The figure shows three views and two pictorial views of one solid part (mm, origin at its lowest corner). Answer the questions. A direction names the side the tool comes from. Round coordinates to 2 decimals unless told otherwise and drop trailing zeros. Write each loop counter-clockwise with the first axis right and the second up, starting at its lowest first coordinate (ties: lowest second). Pieces come first, ordered by that corner, then holes. Notation, with made-up numbers: (44.25, 57.25) - (60.25, 57.25) arc R23 cw to (60.25, 91.25) - close; hole circle Ø3 at (21, 4.5). An arc over 180 degrees is marked (long way). Answer as CSV lines item,"result". Start each with the question number.
Item 1: Which of the six approach directions +Z, -Z, +X, -X, +Y, -Y give full straight-line access (tool end or side, diameter ignored) to the marked faces 1, 2 and 3?
Item 2: For a pull along X with two mould halves and no side action, classify the marked faces 4, 5 and 6 as pulls with the +X half, pulls with the -X half, needs draft (parallel to the pull), parting line crosses it, or undercut.
Item 3: A cutting plane is placed at A-A on z = 3. Determine the outline of the cut face in (x, y).
Item 4: A cutting plane is placed at D-D on z = 0.95. Determine the outline of the cut face in (x, y), and give its area (3 significant figures).
Item 5: Straight lines are drawn through the part: line 1 along X through (y, z) = (15, 1.4); line 2 along X through (y, z) = (15, 2.95); line 3 along Y through (x, z) = (19, 3.2). For each, find the intervals that lie inside material, in ascending order. Write a range as [from, to].
Item 6: A cutting plane is placed at C-C on y = 15. Determine the outline of the cut face in (x, z).
Item 7: Flat-ended cylindrical pins translate along their axes: pin 1 (1 mm diameter, centred on y = 3.5, z = 3.5, fed in from +X); pin 2 (1.7 mm diameter, centred on x = 18, y = 15.5, fed in from +Z). Find the tip coordinate at first contact, or state that the pin passes through.
Item 8: A cutting plane is placed at B-B on x = 4. Determine the outline of the cut face in (y, z), and give its area (3 significant figures).
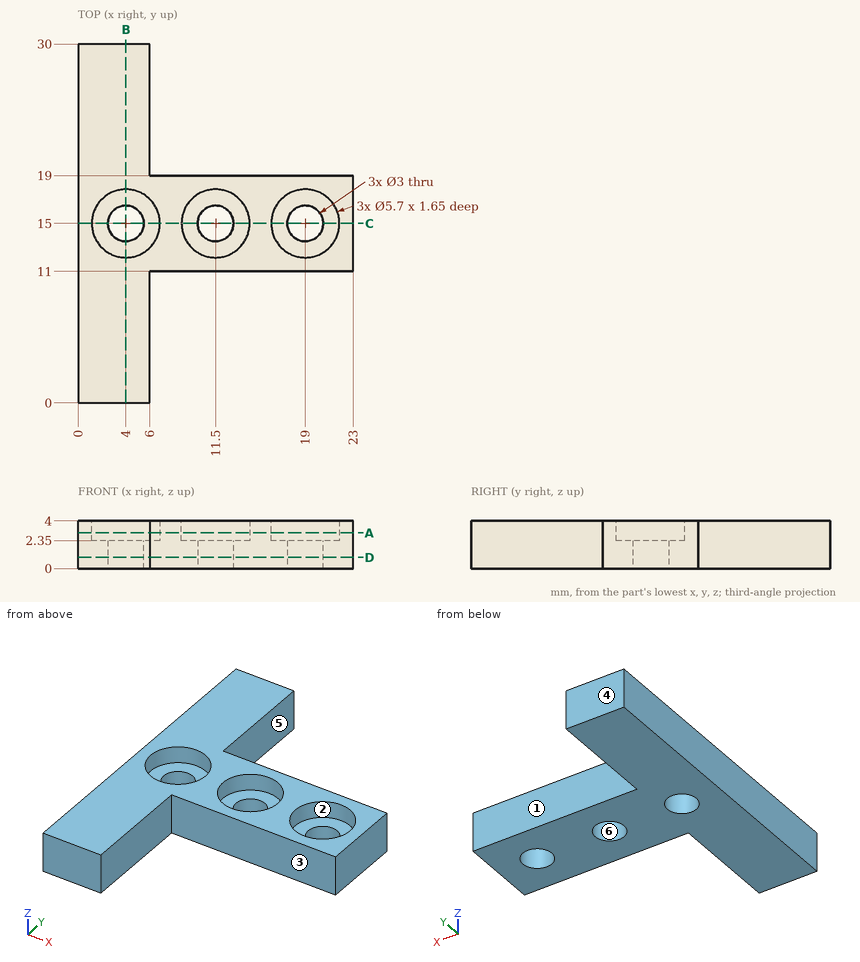
Geometry says:
1,face 1,"+Z, -Z, +X, +Y"
1,face 2,"+Z"
1,face 3,"+Z, -Z, +X, -Y"
2,face 4,"needs draft"
2,face 5,"pulls with the +X half"
2,face 6,"undercut"
3,outline,"(0, 0) - (6, 0) - (6, 11) - (23, 11) - (23, 19) - (6, 19) - (6, 30) - (0, 30) - close; hole circle Ø5.7 at (4, 15); hole circle Ø5.7 at (11.5, 15); hole circle Ø5.7 at (19, 15)"
4,outline,"(0, 0) - (6, 0) - (6, 11) - (23, 11) - (23, 19) - (6, 19) - (6, 30) - (0, 30) - close; hole circle Ø3 at (4, 15); hole circle Ø3 at (11.5, 15); hole circle Ø3 at (19, 15)"
4,area,"295 mm^2"
5,line 1,"x = [0, 2.5], [5.5, 10], [13, 17.5], [20.5, 23]"
5,line 2,"x = [0, 1.15], [6.85, 8.65], [14.35, 16.15], [21.85, 23]"
5,line 3,"y = [11, 12.15], [17.85, 19]"
6,outline,"(0, 0) - (2.5, 0) - (2.5, 2.35) - (1.15, 2.35) - (1.15, 4) - (0, 4) - close; (5.5, 0) - (10, 0) - (10, 2.35) - (8.65, 2.35) - (8.65, 4) - (6.85, 4) - (6.85, 2.35) - (5.5, 2.35) - close; (13, 0) - (17.5, 0) - (17.5, 2.35) - (16.15, 2.35) - (16.15, 4) - (14.35, 4) - (14.35, 2.35) - (13, 2.35) - close; (20.5, 0) - (23, 0) - (23, 4) - (21.85, 4) - (21.85, 2.35) - (20.5, 2.35) - close"
7,pin 1,"stops at x = 6"
7,pin 2,"stops at z = 2.35"
8,outline,"(0, 0) - (13.5, 0) - (13.5, 2.35) - (12.15, 2.35) - (12.15, 4) - (0, 4) - close; (16.5, 0) - (30, 0) - (30, 4) - (17.85, 4) - (17.85, 2.35) - (16.5, 2.35) - close"
8,area,"104 mm^2"
